Check sheet for the modelled part. Datum: model origin and axes. Units: mm. Round coordinates to 2 decimals unless told otherwise and drop trailing zeros. Write each loop counter-clockwise with the first axis right and the second up, starting at its lowest first coordinate (ties: lowest second). Pieces come first, ordered by that corner, then holes. Notation, with made-up numbers: M -12,-31 L 18,-31 A20 cw 18,-1 Z; hole C 75.25,32.25 d11. An arc over 180 degrees is marked long. One line per item, written item: value.
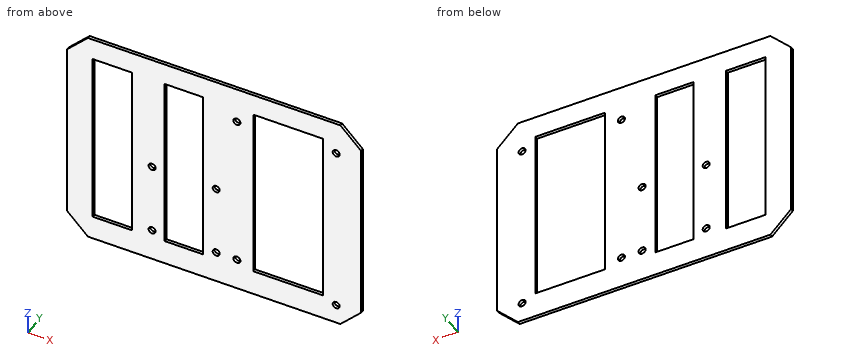
from build123d import *

# Parameters (mm, degrees)
SKETCH1_W           = 142
SKETCH1_H           = 108
BOSS_EXTRUDE1_DEPTH = 1.5
CHAMFER1_SIZE       = 10
CUT_EXTRUDE1_REACH  = 91.215
SKETCH2_R           = 1.7
CUT_EXTRUDE2_REACH  = 91.215
SKETCH3_R           = 1.7
CUT_EXTRUDE3_REACH  = 91.215
SKETCH4_W           = 19.130277945
SKETCH4_H           = 85.726659062
SKETCH4_W_2         = 33.657782249
SKETCH4_H_2         = 85.151312357
SKETCH4_W_3         = 18.55493124
SKETCH4_H_3         = 85.438985709


with BuildPart() as part:
    # Sketch1 → Boss-Extrude1 (new body)
    with BuildSketch(Plane(origin=(0, 0, 0), x_dir=(1, 0, 0), z_dir=(0, 1, 0))):
        Rectangle(SKETCH1_W, SKETCH1_H)
    extrude(amount=BOSS_EXTRUDE1_DEPTH)

    # Chamfer1
    chamfer1_edges = [part.edges().sort_by_distance(p)[0] for p in [
        (71, 0.75, 54),
        (-71, 0.75, 54),
        (-71, 0.75, -54),
        (71, 0.75, -54),
    ]]
    chamfer(chamfer1_edges, length=CHAMFER1_SIZE)

    # Sketch2 → Cut-Extrude1 (cut, up to next)
    with BuildSketch(Plane(origin=(0, 1.5, 0), x_dir=(1, 0, 0), z_dir=(0, 1, 0)), mode=Mode.PRIVATE) as cut_extrude1_sk1:
        with Locations(Location((59, 44.5, 0), (0, 0, 270))):
            Circle(SKETCH2_R)
    cut_extrude1_tool1 = extrude(cut_extrude1_sk1.sketch, amount=-CUT_EXTRUDE1_REACH, mode=Mode.PRIVATE) & part.part
    # Sketch2 → Cut-Extrude1 (cut, up to next)
    with BuildSketch(Plane(origin=(0, 1.5, 0), x_dir=(1, 0, 0), z_dir=(0, 1, 0)), mode=Mode.PRIVATE) as cut_extrude1_sk2:
        with Locations(Location((11, 38.5, 0), (0, 0, 270))):
            Circle(SKETCH2_R)
    cut_extrude1_tool2 = extrude(cut_extrude1_sk2.sketch, amount=-CUT_EXTRUDE1_REACH, mode=Mode.PRIVATE) & part.part
    # Sketch2 → Cut-Extrude1 (cut, up to next)
    with BuildSketch(Plane(origin=(0, 1.5, 0), x_dir=(1, 0, 0), z_dir=(0, 1, 0)), mode=Mode.PRIVATE) as cut_extrude1_sk3:
        with Locations(Location((11, -36.5, 0), (0, 0, 270))):
            Circle(SKETCH2_R)
    cut_extrude1_tool3 = extrude(cut_extrude1_sk3.sketch, amount=-CUT_EXTRUDE1_REACH, mode=Mode.PRIVATE) & part.part
    # Sketch2 → Cut-Extrude1 (cut, up to next)
    with BuildSketch(Plane(origin=(0, 1.5, 0), x_dir=(1, 0, 0), z_dir=(0, 1, 0)), mode=Mode.PRIVATE) as cut_extrude1_sk4:
        with Locations(Location((59, -38, 0), (0, 0, 270))):
            Circle(SKETCH2_R)
    cut_extrude1_tool4 = extrude(cut_extrude1_sk4.sketch, amount=-CUT_EXTRUDE1_REACH, mode=Mode.PRIVATE) & part.part
    add(cut_extrude1_tool1.solids().sort_by_distance((59, 1.5, -44.5))[0], mode=Mode.SUBTRACT)
    add(cut_extrude1_tool2.solids().sort_by_distance((11, 1.5, -38.5))[0], mode=Mode.SUBTRACT)
    add(cut_extrude1_tool3.solids().sort_by_distance((11, 1.5, 36.5))[0], mode=Mode.SUBTRACT)
    add(cut_extrude1_tool4.solids().sort_by_distance((59, 1.5, 38))[0], mode=Mode.SUBTRACT)

    # Sketch3 → Cut-Extrude2 (cut, up to next)
    with BuildSketch(Plane(origin=(0, 1.5, 0), x_dir=(1, 0, 0), z_dir=(0, 1, 0)), mode=Mode.PRIVATE) as cut_extrude2_sk1:
        with Locations(Location((-30, 38.5, 0), (0, 0, 270))):
            Circle(SKETCH3_R)
    cut_extrude2_tool1 = extrude(cut_extrude2_sk1.sketch, amount=-CUT_EXTRUDE2_REACH, mode=Mode.PRIVATE) & part.part
    # Sketch3 → Cut-Extrude2 (cut, up to next)
    with BuildSketch(Plane(origin=(0, 1.5, 0), x_dir=(1, 0, 0), z_dir=(0, 1, 0)), mode=Mode.PRIVATE) as cut_extrude2_sk2:
        with Locations(Location((1, 38.5, 0), (0, 0, 270))):
            Circle(SKETCH3_R)
    cut_extrude2_tool2 = extrude(cut_extrude2_sk2.sketch, amount=-CUT_EXTRUDE2_REACH, mode=Mode.PRIVATE) & part.part
    # Sketch3 → Cut-Extrude2 (cut, up to next)
    with BuildSketch(Plane(origin=(0, 1.5, 0), x_dir=(1, 0, 0), z_dir=(0, 1, 0)), mode=Mode.PRIVATE) as cut_extrude2_sk3:
        with Locations(Location((1, 4, 0), (0, 0, 270))):
            Circle(SKETCH3_R)
    cut_extrude2_tool3 = extrude(cut_extrude2_sk3.sketch, amount=-CUT_EXTRUDE2_REACH, mode=Mode.PRIVATE) & part.part
    # Sketch3 → Cut-Extrude2 (cut, up to next)
    with BuildSketch(Plane(origin=(0, 1.5, 0), x_dir=(1, 0, 0), z_dir=(0, 1, 0)), mode=Mode.PRIVATE) as cut_extrude2_sk4:
        with Locations(Location((-30, 4, 0), (0, 0, 270))):
            Circle(SKETCH3_R)
    cut_extrude2_tool4 = extrude(cut_extrude2_sk4.sketch, amount=-CUT_EXTRUDE2_REACH, mode=Mode.PRIVATE) & part.part
    add(cut_extrude2_tool1.solids().sort_by_distance((-30, 1.5, -38.5))[0], mode=Mode.SUBTRACT)
    add(cut_extrude2_tool2.solids().sort_by_distance((1, 1.5, -38.5))[0], mode=Mode.SUBTRACT)
    add(cut_extrude2_tool3.solids().sort_by_distance((1, 1.5, -4))[0], mode=Mode.SUBTRACT)
    add(cut_extrude2_tool4.solids().sort_by_distance((-30, 1.5, -4))[0], mode=Mode.SUBTRACT)

    # Sketch4 → Cut-Extrude3 (cut, up to next)
    with BuildSketch(Plane(origin=(0, 1.5, 0), x_dir=(1, 0, 0), z_dir=(0, 1, 0)), mode=Mode.PRIVATE) as cut_extrude3_sk1:
        with Locations((-49.192143288, -0.575346705)):
            Rectangle(SKETCH4_W, SKETCH4_H)
    cut_extrude3_tool1 = extrude(cut_extrude3_sk1.sketch, amount=-CUT_EXTRUDE3_REACH, mode=Mode.PRIVATE) & part.part
    # Sketch4 → Cut-Extrude3 (cut, up to next)
    with BuildSketch(Plane(origin=(0, 1.5, 0), x_dir=(1, 0, 0), z_dir=(0, 1, 0)), mode=Mode.PRIVATE) as cut_extrude3_sk2:
        with Locations((35.743414055, -0.863020057)):
            Rectangle(SKETCH4_W_2, SKETCH4_H_2)
    cut_extrude3_tool2 = extrude(cut_extrude3_sk2.sketch, amount=-CUT_EXTRUDE3_REACH, mode=Mode.PRIVATE) & part.part
    # Sketch4 → Cut-Extrude3 (cut, up to next)
    with BuildSketch(Plane(origin=(0, 1.5, 0), x_dir=(1, 0, 0), z_dir=(0, 1, 0)), mode=Mode.PRIVATE) as cut_extrude3_sk3:
        with Locations((-14.67134098, -0.719183381)):
            Rectangle(SKETCH4_W_3, SKETCH4_H_3)
    cut_extrude3_tool3 = extrude(cut_extrude3_sk3.sketch, amount=-CUT_EXTRUDE3_REACH, mode=Mode.PRIVATE) & part.part
    add(cut_extrude3_tool1.solids().sort_by_distance((-49.192143, 1.5, 0.575347))[0], mode=Mode.SUBTRACT)
    add(cut_extrude3_tool2.solids().sort_by_distance((35.743414, 1.5, 0.86302))[0], mode=Mode.SUBTRACT)
    add(cut_extrude3_tool3.solids().sort_by_distance((-14.671341, 1.5, 0.719183))[0], mode=Mode.SUBTRACT)


solid = part.part
Q1. Sectioned sample at D-D on z = -24.5. Enter the section's corners in (x, y).
Completed:
outline: M -71,0 L -58.76,0 L -58.76,1.5 L -71,1.5 Z; M -39.63,0 L -23.95,0 L -23.95,1.5 L -39.63,1.5 Z; M -5.39,0 L 18.91,0 L 18.91,1.5 L -5.39,1.5 Z; M 52.57,0 L 71,0 L 71,1.5 L 52.57,1.5 Z
Q2. Sectioned sample at A-A on y = 1. State how many separate pieces and enclosed holes the cut face has, and give its area (3 significant figures).
Completed:
separate pieces: 1
enclosed holes: 11
area: 8,970 mm^2
Q3. Depth check by flat-ended pin: P1, Ø3, axis at x = 59, z = 38, coming from the +Y side. Enter the tip coordinate at first touch or a pass-through.
Completed:
P1: through
Q4. Sectioned sample at C-C on x = 49.5. Enter the section's corners in (y, z).
Completed:
outline: M 0,-54 L 1.5,-54 L 1.5,-41.71 L 0,-41.71 Z; M 0,43.44 L 1.5,43.44 L 1.5,54 L 0,54 Z
Q5. Scan lines: line 1 (X direction, y = 0.4, z = 24); line 2 (X direction, y = 0.5, z = -4); line 3 (Z direction, x = 26, y = 0.3). Record each from-to range of solid material in increasing order. Write a range as [from, to].
Completed:
line 1: [-71, -58.76], [-39.63, -23.95], [-5.39, 18.91], [52.57, 71]
line 2: [-71, -58.76], [-39.63, -31.7], [-28.3, -23.95], [-5.39, -0.7], [2.7, 18.91], [52.57, 71]
line 3: [-54, -41.71], [43.44, 54]
Q6. Sectioned sample at B-B on z = -38.5. Enter the section's corners in (x, y).
Completed:
outline: M -71,0 L -58.76,0 L -58.76,1.5 L -71,1.5 Z; M -39.63,0 L -31.7,0 L -31.7,1.5 L -39.63,1.5 Z; M -28.3,0 L -23.95,0 L -23.95,1.5 L -28.3,1.5 Z; M -5.39,0 L -0.7,0 L -0.7,1.5 L -5.39,1.5 Z; M 2.7,0 L 9.3,0 L 9.3,1.5 L 2.7,1.5 Z; M 12.7,0 L 18.91,0 L 18.91,1.5 L 12.7,1.5 Z; M 52.57,0 L 71,0 L 71,1.5 L 52.57,1.5 Z
